from build123d import *

# Parameters (mm, degrees)
F2_R     = 0.75
F3_DEPTH = 2


with BuildPart() as f1:
    # F0 (on Front) → F1 (revolve)
    with BuildSketch(Plane.XZ):
        Polygon((-10, 22), (-10, 1020), (-12, 1020), (-12, 20), (-7, 0), (-5, 0), (-10, 20), (0, 20), (0, 22), align=None)
    revolve(axis=Axis((0, 0, 510), (0, 0, 1)))

    # F2 (on face) → F3 (cut, through all)
    with BuildSketch(Plane.XY.offset(22)):
        with Locations((-3.96755, 5.460865)):
            Circle(F2_R)
        with Locations((-6.363961, 6.363961)):
            Circle(F2_R)
        with Locations((-4.5, 7.794229)):
            Circle(F2_R)
        with Locations((-2.085865, 6.419631)):
            Circle(F2_R)
        with Locations((-2.329371, 8.693332)):
            Circle(F2_R)
        with Locations((0, 9)):
            Circle(F2_R)
        with Locations((0, 6.75)):
            Circle(F2_R)
        with Locations((2.085865, 6.419631)):
            Circle(F2_R)
        with Locations((2.329371, 8.693332)):
            Circle(F2_R)
        with Locations((4.5, 7.794229)):
            Circle(F2_R)
        with Locations((6.363961, 6.363961)):
            Circle(F2_R)
        with Locations((3.96755, 5.460865)):
            Circle(F2_R)
        with Locations((5.460865, 3.96755)):
            Circle(F2_R)
        with Locations((7.794229, 4.5)):
            Circle(F2_R)
        with Locations((8.693332, 2.329371)):
            Circle(F2_R)
        with Locations((6.419631, 2.085865)):
            Circle(F2_R)
        with Locations((3.897114, 2.25)):
            Circle(F2_R)
        with Locations((1.948557, 1.125)):
            Circle(F2_R)
        with Locations((2.25, 3.897114)):
            Circle(F2_R)
        with Locations((0, 4.5)):
            Circle(F2_R)
        with Locations((0, 2.25)):
            Circle(F2_R)
        with Locations((-2.25, 3.897114)):
            Circle(F2_R)
        with Locations((-1.948557, 1.125)):
            Circle(F2_R)
        with Locations((-3.897114, 2.25)):
            Circle(F2_R)
        with Locations((-5.460865, 3.96755)):
            Circle(F2_R)
        with Locations((-7.794229, 4.5)):
            Circle(F2_R)
        with Locations((-8.693332, 2.329371)):
            Circle(F2_R)
        with Locations((-6.419631, 2.085865)):
            Circle(F2_R)
        with Locations((-4.5, 0)):
            Circle(F2_R)
        Circle(F2_R)
        with Locations((4.5, 0)):
            Circle(F2_R)
        with Locations((6.75, 0)):
            Circle(F2_R)
        with Locations((9, 0)):
            Circle(F2_R)
        with Locations((1.948557, -1.125)):
            Circle(F2_R)
        with Locations((3.897114, -2.25)):
            Circle(F2_R)
        with Locations((6.419631, -2.085865)):
            Circle(F2_R)
        with Locations((8.693332, -2.329371)):
            Circle(F2_R)
        with Locations((7.794229, -4.5)):
            Circle(F2_R)
        with Locations((6.363961, -6.363961)):
            Circle(F2_R)
        with Locations((5.460865, -3.96755)):
            Circle(F2_R)
        with Locations((3.96755, -5.460865)):
            Circle(F2_R)
        with Locations((4.5, -7.794229)):
            Circle(F2_R)
        with Locations((2.329371, -8.693332)):
            Circle(F2_R)
        with Locations((0, -9)):
            Circle(F2_R)
        with Locations((2.085865, -6.419631)):
            Circle(F2_R)
        with Locations((2.25, -3.897114)):
            Circle(F2_R)
        with Locations((0, -6.75)):
            Circle(F2_R)
        with Locations((0, -4.5)):
            Circle(F2_R)
        with Locations((0, -2.25)):
            Circle(F2_R)
        with Locations((-1.948557, -1.125)):
            Circle(F2_R)
        with Locations((-2.25, -3.897114)):
            Circle(F2_R)
        with Locations((-2.085865, -6.419631)):
            Circle(F2_R)
        with Locations((-2.329371, -8.693332)):
            Circle(F2_R)
        with Locations((-4.5, -7.794229)):
            Circle(F2_R)
        with Locations((-3.96755, -5.460865)):
            Circle(F2_R)
        with Locations((-3.897114, -2.25)):
            Circle(F2_R)
        with Locations((-5.460865, -3.96755)):
            Circle(F2_R)
        with Locations((-6.363961, -6.363961)):
            Circle(F2_R)
        with Locations((-7.794229, -4.5)):
            Circle(F2_R)
        with Locations((-8.693332, -2.329371)):
            Circle(F2_R)
        with Locations((-6.419631, -2.085865)):
            Circle(F2_R)
        with Locations((-6.75, 0)):
            Circle(F2_R)
        with Locations((-9, 0)):
            Circle(F2_R)
    extrude(amount=-F3_DEPTH, mode=Mode.SUBTRACT)


solid = f1.part
Design review of the part built by this model. Coordinates are the model's own, in mm. A direction names the side the tool comes from. Give positions to 0.01 mm unless a question says otherwise; leave off trailing zeros. Loops run counter-clockwise (first coordinate to the right, second up) from the corner with the lowest first, then second, coordinate; pieces in that order, holes last. Notation, with made-up numbers: (3, 53) -> (19, 53) arc R22 cw to (19, 87) -> close; hole circle Ø4 at (19.5, -18). An arc over 180 degrees is marked (long way). One line per question, with ' | ' between items. Start each with the question number.
(1) Draft analysis for pull direction X (two halves, no side actions). For faces 1 (the face through (1.93, 8.7, 7.64)), 2 (the face through (-6.657, -2.096, 7.918)), 3 (the face through (-5, -9, 1020)), state which applies: +X half, -X half, draft (parallel to the pull), parting line (faces both ways), or undercut.
(2) We need section A-A (z = 407). State the section outline as (x, y) points.
(3) For faces 4 (the face through (-1, 0, 22)), 5 (the face through (11.99, -0.53, 513)), 6 (the face through (1, 0, 20)), list the 3-axis set-ups (+Z, -Z, +X, -X, +Y, -Y) from which the entire face can be reached by the end or side of a thin tool; tool diameter is ignored.
(4) Insertion check: P1, Ø5, axis at y = -7.5, z = 745, coming from the +X side; P2, Ø3, axis at y = -8, z = 792, coming from the +X side; P3, Ø1, axis at x = 6.5, z = 379, coming from the -Y side. Each pin has a flat end and moves straight along its axis. Give the tip position at first contact, or say it passes through.
(5) For line 1 (Y direction, x = 0.5, z = 780); line 2 (Y direction, x = -7, z = 427.5), list the stretches that pass through material, from the lowest coordinate up.
The answers:
1) face 1: parting line | face 2: undercut | face 3: draft
2) outline: circle Ø24 at (0, 0); hole circle Ø20 at (0, 0)
3) face 4: +Z | face 5: +Z, -Z | face 6: none
4) P1: stops at x = 10.91 | P2: stops at x = 10.09 | P3: stops at y = -10.39
5) line 1: y = -11.99 to -9.99, 9.99 to 11.99 | line 2: y = -9.75 to -7.14, 7.14 to 9.75
